For this review, take the finished solid that the model builds, in its own axes (mm). Face numbers are marked on the shaded views. A direction names the side the tool comes from. Coordinates: 2 decimals unless noted, no trailing zeros. Loops run counter-clockwise (first coordinate to the right, second up) from the corner with the lowest first, then second, coordinate; pieces in that order, holes last. Notation, with made-up numbers: (-7, 62.25) -> (45, 62.25) arc R11 ccw to (45, 75.25) -> close; hole circle Ø1 at (-12.75, 67.25). An arc over 180 degrees is marked (long way). One line per item, written item: value.
from build123d import *

# Parameters (mm, degrees)
SKETCH_1_R          = 6
SKETCH_1_R_2        = 3.5
EXTRUDE_1_DEPTH     = 2.5
SKETCH_2_R          = 5.5
SKETCH_2_R_2        = 4
CUT_EXTRUDE_1_DEPTH = 0.1
FILLET_1_R          = 0.2


with BuildPart() as part:
    # 草图1 → 凸台-拉伸1 (new, symmetric)
    with BuildSketch(Plane.XY):
        Circle(SKETCH_1_R)
        Circle(SKETCH_1_R_2, mode=Mode.SUBTRACT)
    extrude(amount=EXTRUDE_1_DEPTH, both=True)

    # 草图2 → 切除-拉伸1 (cut)
    with BuildSketch(Plane.XY.offset(2.5)):
        Circle(SKETCH_2_R)
        Circle(SKETCH_2_R_2, mode=Mode.SUBTRACT)
    cut_extrude_1 = extrude(amount=-CUT_EXTRUDE_1_DEPTH, mode=Mode.SUBTRACT)

    # 镜向1: 切除-拉伸1 across plane
    add(cut_extrude_1.mirror(Plane.XY), mode=Mode.SUBTRACT)

    # 圆角1
    # the kernel refuses this fillet: 0.2 mm, written as the material it takes off along each edge
    with BuildSketch(Plane(origin=(0, 0, 2.5), x_dir=(1, 0, 0), z_dir=(0, -1, 0))) as fillet_1_piece_1:
        with BuildLine():
            CenterArc((5.673205081, -0.2), FILLET_1_R, 90, 60)
            Line((5.5, -0.1), (5.496535898, -0.098))
            ThreePointArc((5.496535898, -0.098), (5.496, -0.05), (5.496, 0))
            Line((5.496, 0), (5.5, 0.004))
            Line((5.5, 0.004), (5.673205081, 0.004))
            Line((5.673205081, 0.004), (5.673205081, 0))
        make_face()
    revolve(axis=Axis((0, 0, 2.5), (0, 0, 1)), mode=Mode.SUBTRACT)
    with BuildSketch(Plane(origin=(0, 0, 2.5), x_dir=(1, 0, 0), z_dir=(0, -1, 0))) as fillet_1_piece_2:
        with BuildLine():
            CenterArc((3.826794919, -0.2), FILLET_1_R, 30, 60)
            Line((3.826794919, 0), (3.826794919, 0.004))
            Line((3.826794919, 0.004), (4, 0.004))
            Line((4, 0.004), (4.004, 0))
            ThreePointArc((4.004, 0), (4.004, -0.05), (4.003464102, -0.098))
            Line((4.003464102, -0.098), (4, -0.1))
        make_face()
    revolve(axis=Axis((0, 0, 2.5), (0, 0, 1)), mode=Mode.SUBTRACT)
    with BuildSketch(Plane(origin=(0, 0, -2.5), x_dir=(1, 0, 0), z_dir=(0, -1, 0))) as fillet_1_piece_3:
        with BuildLine():
            CenterArc((3.826794919, 0.2), FILLET_1_R, 270, 60)
            Line((3.826794919, 0), (3.826794919, -0.004))
            Line((3.826794919, -0.004), (4, -0.004))
            Line((4, -0.004), (4.004, 0))
            ThreePointArc((4.004, 0), (4.004, 0.05), (4.003464102, 0.098))
            Line((4.003464102, 0.098), (4, 0.1))
        make_face()
    revolve(axis=Axis((0, 0, -2.5), (0, 0, 1)), mode=Mode.SUBTRACT)
    with BuildSketch(Plane(origin=(0, 0, -2.5), x_dir=(1, 0, 0), z_dir=(0, -1, 0))) as fillet_1_piece_4:
        with BuildLine():
            CenterArc((5.673205081, 0.2), FILLET_1_R, 210, 60)
            Line((5.5, 0.1), (5.496535898, 0.098))
            ThreePointArc((5.496535898, 0.098), (5.496, 0.05), (5.496, 0))
            Line((5.496, 0), (5.5, -0.004))
            Line((5.5, -0.004), (5.673205081, -0.004))
            Line((5.673205081, -0.004), (5.673205081, 0))
        make_face()
    revolve(axis=Axis((0, 0, -2.5), (0, 0, 1)), mode=Mode.SUBTRACT)


solid = part.part
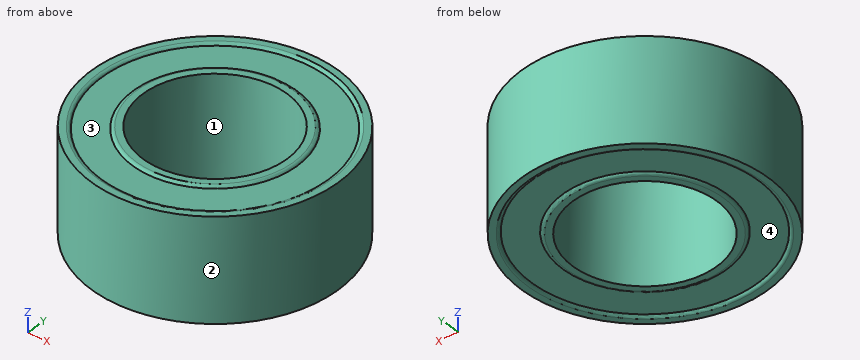
1. Take a section at A-A, the plane y = 0. Give the boundary of the cut face in (x, z).
Return value:
outline: (-6, -2.5) -> (-5.67, -2.5) arc R0.2 ccw to (-5.5, -2.4) -> (-4, -2.4) arc R0.2 ccw to (-3.83, -2.5) -> (-3.5, -2.5) -> (-3.5, 2.5) -> (-3.83, 2.5) arc R0.2 ccw to (-4, 2.4) -> (-5.5, 2.4) arc R0.2 ccw to (-5.67, 2.5) -> (-6, 2.5) -> close; (3.5, -2.5) -> (3.83, -2.5) arc R0.2 ccw to (4, -2.4) -> (5.5, -2.4) arc R0.2 ccw to (5.67, -2.5) -> (6, -2.5) -> (6, 2.5) -> (5.67, 2.5) arc R0.2 ccw to (5.5, 2.4) -> (4, 2.4) arc R0.2 ccw to (3.83, 2.5) -> (3.5, 2.5) -> close
2. For the marked faces 3 and 4, list the 3-axis set-ups (+Z, -Z, +X, -X, +Y, -Y) from which the entire face can be reached by the end or side of a thin tool; tool diameter is ignored.
Return value:
face 3: +Z
face 4: -Z
3. Take a section at C-C, the plane z = -0.05. Give the boundary of the cut face in (x, y).
Return value:
outline: circle Ø12 at (0, 0); hole circle Ø7 at (0, 0)
4. To check wall thickness, follow probe 1 along Y at (x, z) = (0, 1.4); probe 2 along Z at (x, y) = (3.75, -2.5); probe 3 along Y at (x, z) = (-1.5, -1.15). State the ranges of each line that lie inside material, in increasing order. Write a range as from..to.
Return value:
probe 1: y = -6..-3.5, 3.5..6
probe 2: z = -2.4..2.4
probe 3: y = -5.81..-3.16, 3.16..5.81
5. Insertion check: pin 1 Ø1 at (x, z) = (2, 0.5) entering from +Y. The pin has a flat end and moves straight along its axis. Give the tip position at first contact, or say it passes through.
Return value:
pin 1: stops at y = 5.81
6. The part is to be moulded in two halves that separate along X. For the marked faces 1 and 2, say which applies: pulls with the +X half, pulls with the -X half, needs draft (parallel to the pull), parting line crosses it, or undercut.
Return value:
face 1: undercut
face 2: parting line crosses it
